Part model, mm, in its own coordinate system. A direction names the side the tool comes from. Round coordinates to 2 decimals unless told otherwise and drop trailing zeros. Loops run counter-clockwise (first coordinate to the right, second up) from the corner with the lowest first, then second, coordinate; pieces in that order, holes last. Notation, with made-up numbers: M 89,-10 L 109,-10 A33 ccw 109,23 Z; hole C 54.5,30.5 d9. An arc over 180 degrees is marked long. Put each result on its own line as item: value. Start each with the question number.
1) Slice it at D-D on y = 2. Give the cut face in (x, z), then the cut area to 3 significant figures.
2) Slice it at A-A on x = 0. Give the cut face in (y, z) (1 decimal), then the cut area to 3 significant figures.
3) Probe line 1 along Y through (x, z) = (-1.25, 6.75); line 2 along X through (y, z) = (2.25, 4). List the from-to ranges inside material, lowest first.
4) Which spindle directions (+Z, -Z, +X, -X, +Y, -Y) get a long thin tool onto all of the face, cutting with end or side? Do faces 1 (the flat face through (1.588, 0, 11)), 2 (the flat face through (0.794, 2, 4)), 3 (the flat face through (1, -1, 0)), 4 (the flat face through (2, 0.794, 4)). Say none if no direction does.
5) Pull direction Y, two halves, no side cores. Call faces 5 (the cylindrical face through (-0.41, 3.15, 5.48)), 6 (the flat face through (-1.588, 0, 11)), 7 (the flat face through (0, 2.381, 4)): +Y half, -Y half, draft (parallel to the pull), parting line (faces both ways), or undercut.
6) Drop flat-ended pins along their axis: pin 1 Ø0.8 at (y, z) = (-1.5, 2) entering from -X; pin 2 Ø0.5 at (x, z) = (2, 3) entering from +Y; pin 3 Ø1.7 at (y, z) = (1.5, 4.5) entering from -X. Give the stop position or say it passes through.
```python
from build123d import *

# Parameters (mm, degrees)
F0_R     = 3.175
F1_DEPTH = 14.2875
F2_R     = 3.175
F4_DEPTH = 12.7
F5_W     = 1.5875
F5_H     = 1.5875
F6_DEPTH = 7.9375


with BuildPart() as f1:
    # F0 (on Top) → F1 (new body)
    with BuildSketch(Plane.XY):
        Circle(F0_R)
    extrude(amount=F1_DEPTH)

    # F2
    f2_edges = [f1.edges().sort_by_distance(p)[0] for p in [
        (-3.175, 0, 14.2875),
    ]]
    fillet(f2_edges, radius=F2_R)

    # F3 (on Front) → F4 (cut, symmetric)
    with BuildSketch(Plane.XZ):
        Polygon((-1.5875, 7.9375), (0, 7.9375), (1.5875, 7.9375), (1.5875, 14.9094229564), (-1.5875, 14.9094229564), align=None)
    extrude(amount=F4_DEPTH, both=True, mode=Mode.SUBTRACT)

    # F5 (on face) → F6 (cut)
    with BuildSketch(Plane(origin=(0, 0, 0), x_dir=(1, 0, 0), z_dir=(0, 0, -1))):
        with Locations((-1.5875, 0)):
            Rectangle(F5_W, F5_H)
        with Locations((0, 1.5875)):
            Rectangle(F5_W, F5_H)
        Rectangle(F5_W, F5_H)
        with Locations((1.5875, 0)):
            Rectangle(F5_W, F5_H)
        with Locations((0, -1.5875)):
            Rectangle(F5_W, F5_H)
    extrude(amount=-F6_DEPTH, mode=Mode.SUBTRACT)


solid = f1.part
```
Recorded:
1. outline: M -2.47,0 L -0.79,0 L -0.79,7.94 L -1.59,7.94 L -1.59,13 A2.47 ccw -2.47,11.11 Z; M 0.79,0 L 2.47,0 L 2.47,11.11 A2.47 ccw 1.59,13 L 1.59,7.94 L 0.79,7.94 Z
1. area: 34.4 mm2
2. outline: M -3.2,0 L -2.4,0 L -2.4,7.9 L -3.2,7.9 Z; M 2.4,0 L 3.2,0 L 3.2,7.9 L 2.4,7.9 Z
2. area: 12.6 mm2
3. line 1: y = -2.92 to -0.79, 0.79 to 2.92
3. line 2: x = -2.24 to -0.79, 0.79 to 2.24
4. face 1: +Z, +Y, -Y
4. face 2: +Z, -Z
4. face 3: -Z, +X, -X, +Y, -Y
4. face 4: -Z
5. face 5: parting line
5. face 6: draft
5. face 7: undercut
6. pin 1: stops at x = -2.98
6. pin 2: stops at y = 2.65
6. pin 3: stops at x = -3.11
